```python
from build123d import *

# Parameters (mm, degrees)
F0_R     = 6.1
F0_R_2   = 4.4
F0_R_3   = 2.75
F0_R_4   = 1.45
F1_DEPTH = 2.35
F2_DEPTH = 5.55
F3_R     = 0.8
F4_DEPTH = 2.35
F6_R     = 4.5
F6_R_2   = 3.4
F6_R_3   = 2.9
F7_DEPTH = 0.7


# Not quite as in the source:
# - a pattern or mirror of a feature is missing from the dataset's text; its kind, count and spacing are read off the source's solid


with BuildPart() as f1:
    # F0 (on Top) → F1 (new body)
    with BuildSketch(Plane.XY):
        Circle(F0_R)
        Circle(F0_R_2, mode=Mode.SUBTRACT)
        Circle(F0_R_2)
        Circle(F0_R_3, mode=Mode.SUBTRACT)
        Circle(F0_R_3)
        Circle(F0_R_4, mode=Mode.SUBTRACT)
    extrude(amount=F1_DEPTH)

    # F0 (on Top) → F2 (join)
    with BuildSketch(Plane.XY):
        Circle(F0_R_2)
        Circle(F0_R_3, mode=Mode.SUBTRACT)
    extrude(amount=F2_DEPTH)

    # F3 (on Top) → F4 (join, through all)
    with BuildSketch(Plane.XY):
        with BuildLine():
            Line((-2.5739052597, 16.8674394022), (-4.375, 4.2508087466))
            ThreePointArc((-4.375, 4.2508087466), (0, 6.1), (4.375, 4.2508087466))
            Line((4.375, 4.2508087466), (2.5739052597, 16.8674394022))
            ThreePointArc((2.5739052597, 16.8674394022), (0, 19.1), (-2.5739052597, 16.8674394022))
        make_face()
        with Locations((0, 7.5)):
            Circle(F3_R, mode=Mode.SUBTRACT)
        with Locations((0, 10.5)):
            Circle(F3_R, mode=Mode.SUBTRACT)
        with Locations((0, 13.5)):
            Circle(F3_R, mode=Mode.SUBTRACT)
        with Locations((0, 16.5)):
            Circle(F3_R, mode=Mode.SUBTRACT)
    f4 = extrude(amount=F4_DEPTH)

    # F4_copies: F4 across plane
    add(f4.mirror(Plane(origin=(0, 0, 0), x_dir=(0, 0, -1), z_dir=(0, -1, 0))))

    # F6 (on face) → F7 (cut)
    with BuildSketch(Plane(origin=(0, 0, 0), x_dir=(1, 0, 0), z_dir=(0, 0, -1))):
        Circle(F6_R)
        Circle(F6_R_2, mode=Mode.SUBTRACT)
        Circle(F6_R_3)
    extrude(amount=-F7_DEPTH, mode=Mode.SUBTRACT)


solid = f1.part
```
Work out the finished part from the listing and answer in its coordinate system (mm). A direction names the side the tool comes from. Give positions to 0.01 mm unless a question says otherwise; leave off trailing zeros. Order: outer loops, then holes, each group sorted by start corner. A loop starts at its lowest first (then second) coordinate and runs counter-clockwise, first axis right, second up.
1. Section A-A, the plane y = 0 is taken. Determine the outline of the cut face in (x, z), and give its area (3 significant figures).
Result sheet:
outline: (-6.1, 0) - (-4.5, 0) - (-4.5, 0.7) - (-3.4, 0.7) - (-3.4, 0) - (-2.9, 0) - (-2.9, 0.7) - (-1.45, 0.7) - (-1.45, 2.35) - (-2.75, 2.35) - (-2.75, 5.55) - (-4.4, 5.55) - (-4.4, 2.35) - (-6.1, 2.35) - close; (1.45, 0.7) - (2.9, 0.7) - (2.9, 0) - (3.4, 0) - (3.4, 0.7) - (4.5, 0.7) - (4.5, 0) - (6.1, 0) - (6.1, 2.35) - (4.4, 2.35) - (4.4, 5.55) - (2.75, 5.55) - (2.75, 2.35) - (1.45, 2.35) - close
area: 28.8 mm2
2. Section B-B, the plane z = 3.3 is taken. Determine the outline of the cut face in (x, y), and give its area (3 significant figures).
Result sheet:
outline: circle Ø8.8 at (0, 0); hole circle Ø5.5 at (0, 0)
area: 37.1 mm2
3. For faces 1 (the flat face through (0, 5, 0)), 2 (the flat face through (1.2, -1.2, 2.35)), 3 (the cylindrical face through (-2.9, -0.1, 0.3)), determine the directions among +Z, -Z, +X, -X, +Y, -Y from which every point of the face is accessible in a straight line to the end or side of a thin tool.
Result sheet:
face 1: -Z, +X, -X, +Y, -Y
face 2: +Z
face 3: -Z
4. Each of these flat-tipped pins is pushed along its axis until it touches: P1, Ø2, axis at x = 0, y = 16.5, coming from the +Z side; P2, Ø3.5, axis at x = 0, y = 0, coming from the -Z side; P3, Ø3, axis at y = -14, z = 3, coming from the -X side. Where does it stop, or does it pass through?
Result sheet:
P1: stops at z = 2.35
P2: stops at z = 0.7
P3: stops at x = -3.18
5. The mould has two halves that part along X. Classify faces 4 (the cylindrical face through (-0.596, -2.685, 3.928)), 5 (the cylindrical face through (-0.104, -8.293, 1.159)), 6 (the cylindrical face through (-6.1, 0.1, 1.2)), 7 (the cylindrical face through (4.197, 1.322, 3.928)): released by +X, released by -X, zero draft, split by the parting line, or undercut.
Result sheet:
face 4: undercut
face 5: undercut
face 6: released by -X
face 7: split by the parting line
6. Straight lines are drawn through the part: L1, parallel to Y at x = 0, z = 3.6; L2, parallel to Y at x = 1, z = 2.8; L3, parallel to Z at x = -4.25, y = -2. For each, find the intervals that lie inside material, in ascending order.
Result sheet:
L1: y = -4.4 to -2.75, 2.75 to 4.4
L2: y = -4.28 to -2.56, 2.56 to 4.28
L3: z = 0 to 2.35
7. Section D-D, the plane y = -16.5 is taken. Determine the outline of the cut face in (x, z).
Result sheet:
outline: (-2.63, 0) - (-0.8, 0) - (-0.8, 2.35) - (-2.63, 2.35) - close; (0.8, 0) - (2.63, 0) - (2.63, 2.35) - (0.8, 2.35) - close
8. Section C-C, the plane x = 0 is taken. Give the number of separate pieces and of enclosed holes in the cut face, and give its area (3 significant figures).
Result sheet:
separate pieces: 10
enclosed holes: 0
area: 59.9 mm2
